Here's how the part is built. I have some questions about the finished solid (model axes, mm). Face numbers are marked on the shaded views. A direction names the side the tool comes from. Coordinates: 2 decimals unless noted, no trailing zeros. Write each loop counter-clockwise with the first axis right and the second up, starting at its lowest first coordinate (ties: lowest second). Pieces come first, ordered by that corner, then holes. Notation, with made-up numbers: (-19.5, 30.5) -> (-15.5, 30.5) arc R35 ccw to (-15.5, 63.5) -> close; hole circle Ø7 at (13, 32). An arc over 180 degrees is marked (long way). Put each result on its own line as item: value.
```python
from build123d import *

# Parameters (mm, degrees)
SKETCH1_W           = 40
SKETCH1_H           = 55
BOSS_EXTRUDE1_DEPTH = 5
SKETCH1_3_W         = 40
SKETCH1_3_H         = 5
BOSS_EXTRUDE2_DEPTH = 25
SKETCH2_R           = 4
CUT_EXTRUDE1_DEPTH  = 6


with BuildPart() as part:
    # Sketch1 → Boss-Extrude1 (new body)
    with BuildSketch(Plane.XY):
        with Locations((20, 27.5)):
            Rectangle(SKETCH1_W, SKETCH1_H)
    extrude(amount=BOSS_EXTRUDE1_DEPTH)

    # Sketch1<3> → Boss-Extrude2 (add)
    with BuildSketch(Plane.XY):
        with Locations((20, -2.5)):
            Rectangle(SKETCH1_3_W, SKETCH1_3_H)
    extrude(amount=BOSS_EXTRUDE2_DEPTH)

    # Sketch2 → Cut-Extrude1 (cut, through all)
    with BuildSketch(Plane.XY.offset(5)):
        with Locations((20, 35)):
            Circle(SKETCH2_R)
    extrude(amount=-CUT_EXTRUDE1_DEPTH, mode=Mode.SUBTRACT)


solid = part.part
```
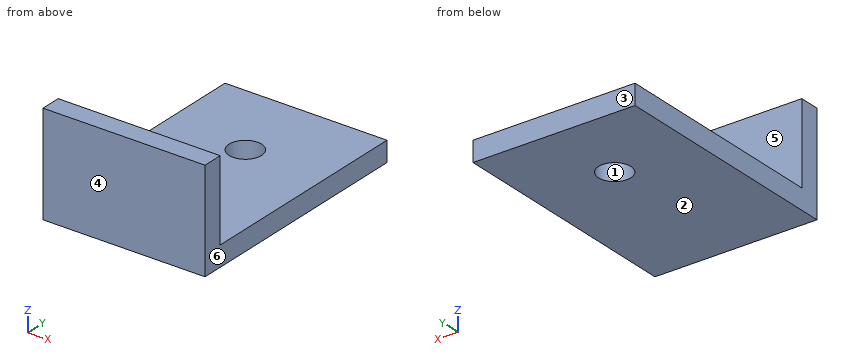
Item 1: Imagine slicing it at D-D on y = 23.5. Write out the boundary of the cut face in (x, z).
Output:
outline: (0, 0) -> (40, 0) -> (40, 5) -> (0, 5) -> close
Item 2: Imagine slicing it at A-A on y = 35. Write out the boundary of the cut face in (x, z), then the cut area to 3 significant figures.
Output:
outline: (0, 0) -> (16, 0) -> (16, 5) -> (0, 5) -> close; (24, 0) -> (40, 0) -> (40, 5) -> (24, 5) -> close
area: 160 mm²
Item 3: For P1, Ø6, axis at x = 15.5, z = 12, coming from the +Y side; P2, Ø6.5, axis at x = 20, y = 35, coming from the +Z side, each with a flat end and sliding along its axis, tell me the tip position at first contact or that it passes through.
Output:
P1: stops at y = 0
P2: passes through
Item 4: Imagine slicing it at C-C on x = 7. Write out the boundary of the cut face in (y, z).
Output:
outline: (-5, 0) -> (55, 0) -> (55, 5) -> (0, 5) -> (0, 25) -> (-5, 25) -> close
Item 5: Imagine slicing it at B-B on x = 20. Write out the boundary of the cut face in (y, z).
Output:
outline: (-5, 0) -> (31, 0) -> (31, 5) -> (0, 5) -> (0, 25) -> (-5, 25) -> close; (39, 0) -> (55, 0) -> (55, 5) -> (39, 5) -> close
Item 6: Which directions (+Z, -Z, +X, -X, +Y, -Y) give clear straight access to the entire face, cutting with the end or side of a thin tool? Please do the marked faces 5 and 6.
Output:
face 5: +Z, +X, -X, +Y
face 6: +Z, -Z, +X, +Y, -Y
Item 7: Please list where these lines run through material, in increasing order: line 1 along Y through (x, z) = (20, 1.75); line 2 along Y through (x, z) = (32, 8); line 3 along Z through (x, y) = (37, 48). Write a range as from..to.
Output:
line 1: y = -5..31, 39..55
line 2: y = -5..0
line 3: z = 0..5
Item 8: If we mould it in two halves opening along Y, with no side actions, what happens to the marked faces 1, 2, 3 and 4? For each: released by +Y, released by -Y, zero draft, split by the parting line, or undercut.
Output:
face 1: undercut
face 2: zero draft
face 3: released by +Y
face 4: released by -Y
